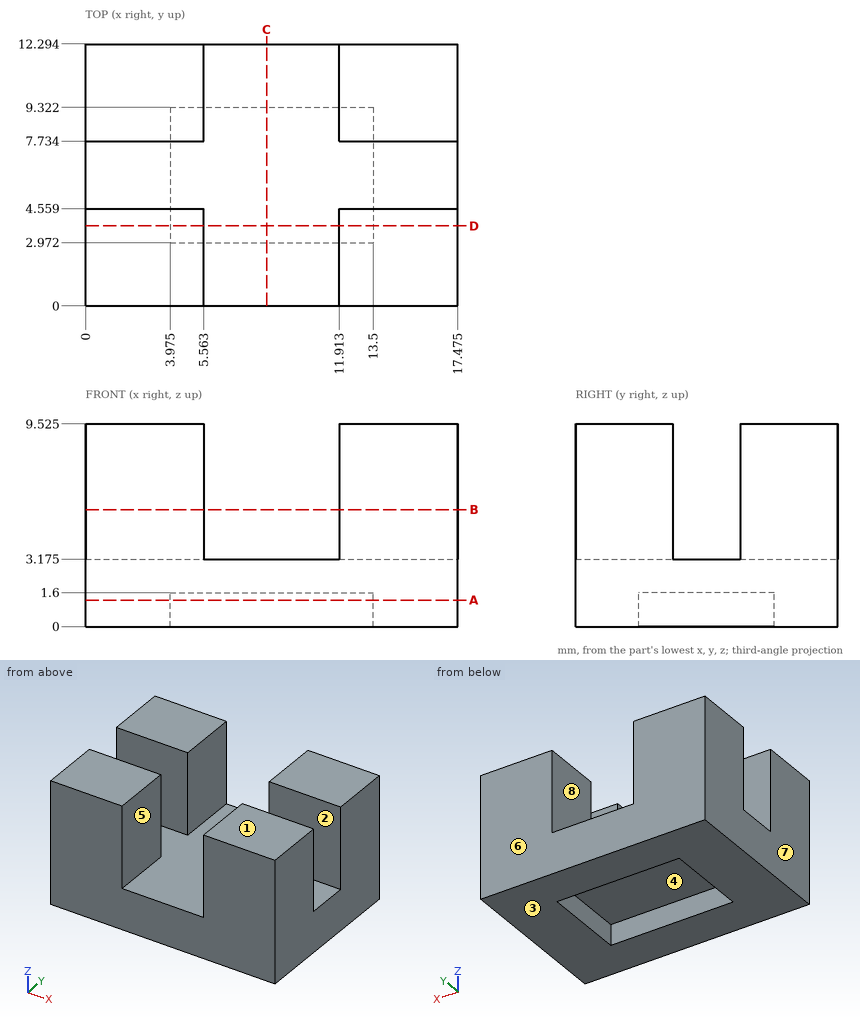
Check sheet for the drawn part. Datum: minimum x, y, z corner. Units: mm. A direction names the side the tool comes from. Round coordinates to 2 decimals unless told otherwise and drop trailing zeros. Order: outer loops, then holes, each group sorted by start corner. A loop starts at its lowest first (then second) coordinate and runs counter-clockwise, first axis right, second up. Notation, with made-up numbers: (85.25, 78) -> (102.25, 78) arc R21 cw to (102.25, 91) -> close; hole circle Ø4 at (-4.5, -16.5). An arc over 180 degrees is marked (long way). Return JSON: item names as keys, results as strings. Group by question number.
Q1. Section check C-C, the plane x = 8.5. Record the boundary of the cut face in (y, z) (1 decimal).
Q2. Release check for a two-part mould opening along X. For the marked faces 6, 7 and 8 record: released by +X, released by -X, zero draft, split by the parting line, or undercut.
Q3. Gauge pin test, flat ends, axial feed: pin 1 (0.8 mm diameter, centred on x = 11, z = 0.5, fed in from -Y); pin 2 (1.5 mm diameter, centred on x = 6.5, y = 6, fed in from +Z) (3 decimals); pin 3 (1.9 mm diameter, centred on x = 10, y = 7, fed in from -Z). Record the tip position at first contact, or that the pin passes through.
Q4. Section check B-B, the plane z = 5.5. Record the boundary of the cut face in (x, y) (1 decimal).
Q5. Section check A-A, the plane z = 1.25. Record the boundary of the cut face in (x, y) (1 decimal), plus the area to 3 significant figures.
Q6. Material ranges on probe 1 along Y at (x, z) = (3.5, 3.25) (1 decimal); probe 2 along Y at (x, z) = (4.75, 1); probe 3 along X at (y, z) = (9, 3.75) (1 decimal), recorded low to high. Write a range as from..to.
Q7. Section check D-D, the plane y = 3.75. Record the boundary of the cut face in (x, z) (1 decimal).
Q8. Tool access check on the marked faces 1, 2, 3, 4 and 5. Record the directions out of +Z, -Z, +X, -X, +Y, -Y that give a thin tool (end or side, any length) a straight path to the whole face; none if there is none.
Numbers:
{
 "1": {"outline": "(0, 0) -> (3, 0) -> (3, 1.6) -> (9.3, 1.6) -> (9.3, 0) -> (12.3, 0) -> (12.3, 3.2) -> (0, 3.2) -> close"},
 "2": {"face 6": "zero draft", "face 7": "released by -X", "face 8": "undercut"},
 "3": {"pin 1": "y = 0", "pin 2": "z = 3.175", "pin 3": "z = 1.6"},
 "4": {"outline": "(0, 0) -> (5.6, 0) -> (5.6, 4.6) -> (0, 4.6) -> close; (0, 7.7) -> (5.6, 7.7) -> (5.6, 12.3) -> (0, 12.3) -> close; (11.9, 0) -> (17.5, 0) -> (17.5, 4.6) -> (11.9, 4.6) -> close; (11.9, 7.7) -> (17.5, 7.7) -> (17.5, 12.3) -> (11.9, 12.3) -> close"},
 "5": {"outline": "(0, 0) -> (17.5, 0) -> (17.5, 12.3) -> (0, 12.3) -> close; hole (4, 3) -> (13.5, 3) -> (13.5, 9.3) -> (4, 9.3) -> close", "area": "154 mm^2"},
 "6": {"probe 1": "0..4.6, 7.7..12.3", "probe 2": "0..2.97, 9.32..12.29", "probe 3": "0..5.6, 11.9..17.5"},
 "7": {"outline": "(0, 0) -> (4, 0) -> (4, 1.6) -> (13.5, 1.6) -> (13.5, 0) -> (17.5, 0) -> (17.5, 9.5) -> (11.9, 9.5) -> (11.9, 3.2) -> (5.6, 3.2) -> (5.6, 9.5) -> (0, 9.5) -> close"},
 "8": {"face 1": "+Z, +X, -X, +Y, -Y", "face 2": "+Z, +X, -X", "face 3": "-Z, +X, -X, +Y, -Y", "face 4": "-Z", "face 5": "+Z, +Y, -Y"}
}
